```python
from build123d import *

# Parameters (mm, degrees)
F0_W     = 127
F0_H     = 112
F1_DEPTH = 3
F2_W     = 3.05
F2_H     = 10
F2_R     = 1.575
F2_W_2   = 20
F2_H_2   = 3.05
F3_DEPTH = 3
F4_R     = 3


with BuildPart() as f1:
    # F0 (on Top) → F1 (new body)
    with BuildSketch(Plane.XY):
        Rectangle(F0_W, F0_H)
    extrude(amount=F1_DEPTH)

    # F2 (on face) → F3 (cut, through all)
    with BuildSketch(Plane.XY.offset(3)):
        with Locations((-58.025, 25)):
            Rectangle(F2_W, F2_H)
        with Locations((-58.025, -25)):
            Rectangle(F2_W, F2_H)
        with Locations((-58.025, 0)):
            Circle(F2_R)
        with Locations((58.025, -25)):
            Rectangle(F2_W, F2_H)
        with Locations((58.025, 25)):
            Rectangle(F2_W, F2_H)
        with Locations((58.025, 0)):
            Circle(F2_R)
        with Locations((-35, -51.525)):
            Rectangle(F2_W_2, F2_H_2)
        with Locations((35, -51.525)):
            Rectangle(F2_W_2, F2_H_2)
        with Locations((0, -51.525)):
            Circle(F2_R)
        with Locations((-35, 51.525)):
            Rectangle(F2_W_2, F2_H_2)
        with Locations((35, 51.525)):
            Rectangle(F2_W_2, F2_H_2)
        with Locations((0, 51.525)):
            Circle(F2_R)
    extrude(amount=-F3_DEPTH, mode=Mode.SUBTRACT)

    # F4
    f4_edges = [f1.edges().sort_by_distance(p)[0] for p in [
        (63.5, -56, 1.5),
        (-63.5, -56, 1.5),
        (-63.5, 56, 1.5),
        (63.5, 56, 1.5),
    ]]
    fillet(f4_edges, radius=F4_R)


solid = f1.part
```
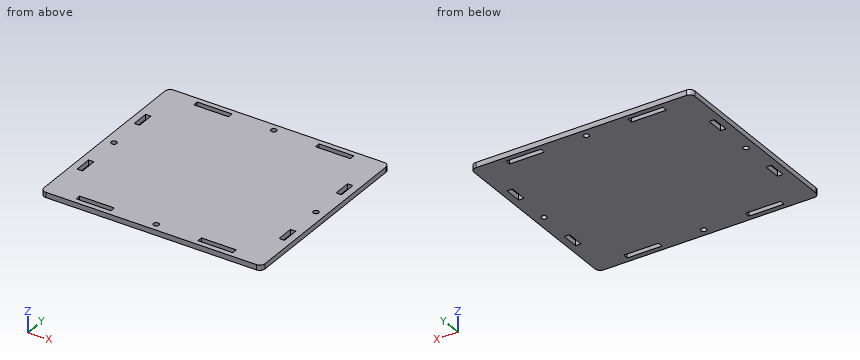
Check sheet for the modelled part. Datum: model origin and axes. Units: mm. Round coordinates to 2 decimals unless told otherwise and drop trailing zeros. Order: outer loops, then holes, each group sorted by start corner. A loop starts at its lowest first (then second) coordinate and runs counter-clockwise, first axis right, second up. Notation, with made-up numbers: (23.25, 29.25) -> (78.25, 29.25) arc R25 cw to (78.25, 50.25) -> close; hole circle Ø3 at (62.5, 4). An arc over 180 degrees is marked (long way). One line per item, written item: value. Start each with the question number.
Q1. Cross-section at C-C (z = 1.25). Give the number of separate pieces and of enclosed holes in the cut face, and give its area (3 significant figures).
Q2. Thickness scan on line 1 (Y direction, x = -27, z = 1.85); line 2 (Y direction, x = 0, z = 0.8); line 3 (X direction, y = -23, z = 1.3). Record the ranges inside material, lowest first.
Q3. Gauge pin test, flat end, axial feed: pin 1 Ø3 at (x, y) = (-58.025, 0) entering from -Z. Record the tip position at first contact, or that the pin passes through.
Q4. Cross-section at B-B (y = 0). Record the boundary of the cut face in (x, z).
Q5. Cross-section at A-A (x = 0). Record the boundary of the cut face in (y, z).
Completed:
1. separate pieces: 1
1. enclosed holes: 12
1. area: 13,800 mm²
2. line 1: y = -56 to -53.05, -50 to 50, 53.05 to 56
2. line 2: y = -56 to -53.1, -49.95 to 49.95, 53.1 to 56
2. line 3: x = -63.5 to -59.55, -56.5 to 56.5, 59.55 to 63.5
3. pin 1: passes through
4. outline: (-63.5, 0) -> (-59.6, 0) -> (-59.6, 3) -> (-63.5, 3) -> close; (-56.45, 0) -> (56.45, 0) -> (56.45, 3) -> (-56.45, 3) -> close; (59.6, 0) -> (63.5, 0) -> (63.5, 3) -> (59.6, 3) -> close
5. outline: (-56, 0) -> (-53.1, 0) -> (-53.1, 3) -> (-56, 3) -> close; (-49.95, 0) -> (49.95, 0) -> (49.95, 3) -> (-49.95, 3) -> close; (53.1, 0) -> (56, 0) -> (56, 3) -> (53.1, 3) -> close
